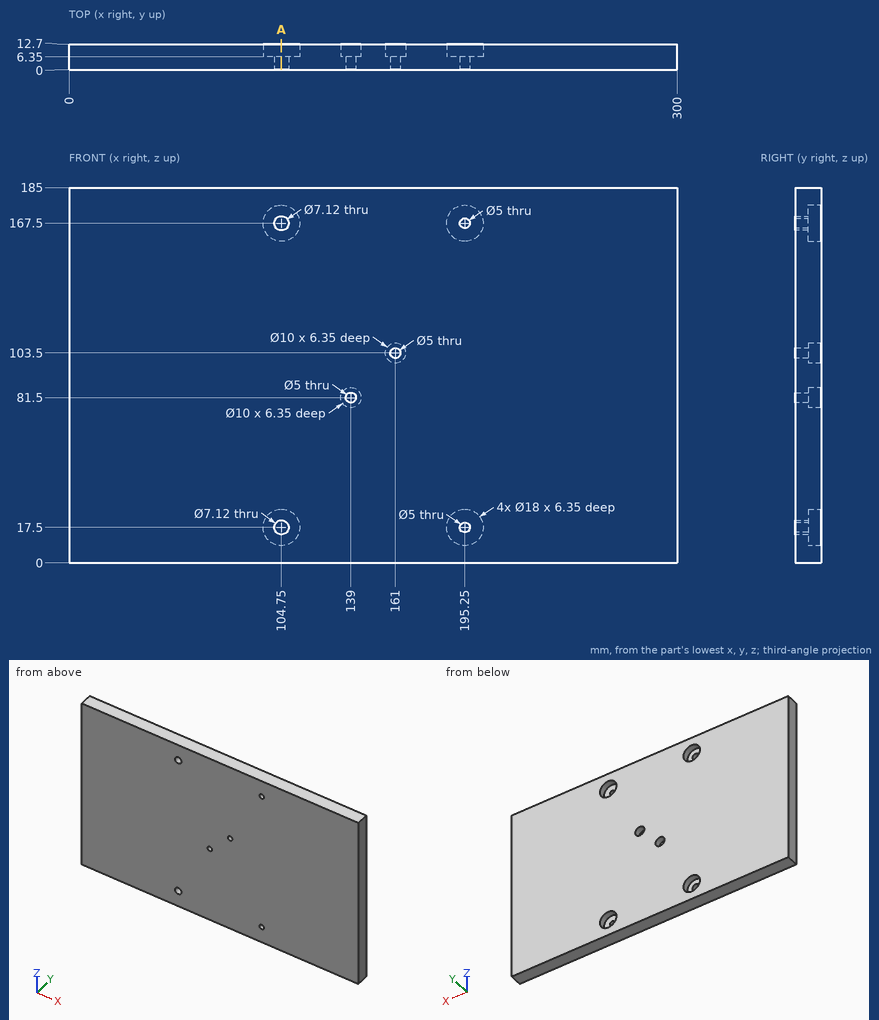
Design review of the part shown in the three views and the two pictorial views. Dimensions are in mm from the part's minimum x, y and z. Coordinates: 2 decimals unless noted, no trailing zeros. Write each loop counter-clockwise with the first axis right and the second up, starting at its lowest first coordinate (ties: lowest second). Pieces come first, ordered by that corner, then holes.
1) To check wall thickness, follow probe 1 along Z at (x, y) = (195.25, 3.75); probe 2 along Z at (x, y) = (105, 10); probe 3 along X at (y, z) = (8.75, 103.5). State the ranges of each line that lie inside material, in increasing order.
2) Clearance check with a flat-ended pin moving along its axis: pin 1 Ø11 at (x, z) = (104.75, 17.5) entering from +Y. State where the tip first meets the part, or that it passes through.
3) We need section A-A on x = 104.75. State the section outline as (y, z) points.
Answer list:
1. probe 1: z = 0 to 15, 20 to 165, 170 to 185
1. probe 2: z = 0 to 8.5, 26.5 to 158.5, 176.5 to 185
1. probe 3: x = 0 to 156, 166 to 300
2. pin 1: stops at y = 6.35
3. outline: (0, 0) - (12.7, 0) - (12.7, 8.5) - (6.35, 8.5) - (6.35, 13.94) - (0, 13.94) - close; (0, 21.06) - (6.35, 21.06) - (6.35, 26.5) - (12.7, 26.5) - (12.7, 158.5) - (6.35, 158.5) - (6.35, 163.94) - (0, 163.94) - close; (0, 171.06) - (6.35, 171.06) - (6.35, 176.5) - (12.7, 176.5) - (12.7, 185) - (0, 185) - close
